CAD build for the part. Positions are in the model's coordinates, mm. Face numbers are marked on the shaded views. A direction names the side the tool comes from. Give positions to 0.01 mm unless a question says otherwise; leave off trailing zeros. Loops run counter-clockwise (first coordinate to the right, second up) from the corner with the lowest first, then second, coordinate; pieces in that order, holes last.
```python
from build123d import *

# Parameters (mm, degrees)
F1_DEPTH = 8


with BuildPart() as f1:
    # F0 (on Front) → F1 (new body)
    with BuildSketch(Plane.XZ):
        Polygon((-12, 6.928203), (-12, -6.928203), (0, -13.856406), (12, -6.928203), (12, 6.928203), (0, 13.856406), align=None)
    extrude(amount=F1_DEPTH)

    # F2 (on Right) → F3 (revolve)
    with BuildSketch(Plane.YZ):
        Polygon((1.602202, 3.686891), (0, 3.686891), (0, 0), (23.874549, 0), (23.874549, 3.686891), align=None)
    revolve(axis=Axis((0, 11.937275, 0), (0, 1, 0)))


solid = f1.part
```
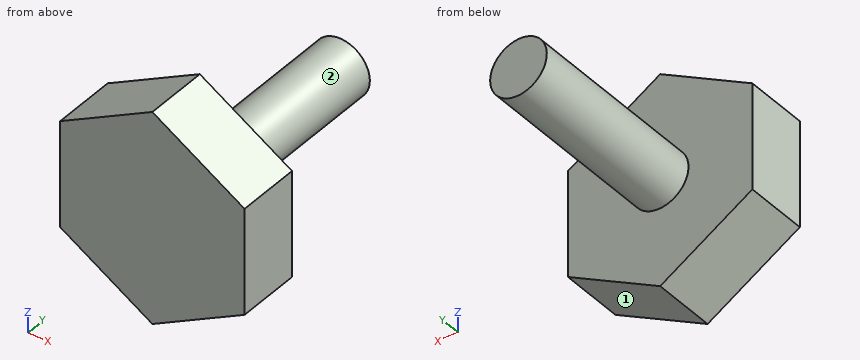
1. Saw through at A-A, the plane z = 0. List the corners of the cut face in (x, y), and give its area (3 significant figures).
Responses:
outline: (-12, -8) - (12, -8) - (12, 0) - (3.69, 0) - (3.69, 23.87) - (-3.69, 23.87) - (-3.69, 0) - (-12, 0) - close
area: 368 mm2
2. Drop flat-ended pins along their axis: pin 1 (12 mm diameter, centred on x = 2.5, z = 3, fed in from +Y); pin 2 (4 mm diameter, centred on x = 3.5, y = 2.5, fed in from +Z); pin 3 (5 mm diameter, centred on x = -2.5, y = 6, fed in from +Z). Give the stop position or say it passes through.
Responses:
pin 1: stops at y = 23.87
pin 2: stops at z = 3.37
pin 3: stops at z = 3.69
3. Saw through at C-C, the plane x = -5.25. List the corners of the cut face in (y, z), and give its area (3 significant figures).
Responses:
outline: (-8, -10.83) - (0, -10.83) - (0, 10.83) - (-8, 10.83) - close
area: 173 mm2
4. Probe line 1 along Y through (x, z) = (-8.75, 1.25); line 2 along Z through (x, y) = (-0.25, 8.5); line 3 along X through (y, z) = (6.5, -3). List the from-to ranges inside material, lowest first.
Responses:
line 1: y = -8 to 0
line 2: z = -3.68 to 3.68
line 3: x = -2.14 to 2.14
5. Saw through at D-D, the plane z = 11.75. List the corners of the cut face in (x, y).
Responses:
outline: (-3.65, -8) - (3.65, -8) - (3.65, 0) - (-3.65, 0) - close
6. Saw through at B-B, the plane x = -1.5. List the corners of the cut face in (y, z).
Responses:
outline: (-8, -12.99) - (0, -12.99) - (0, -3.37) - (23.87, -3.37) - (23.87, 3.37) - (0, 3.37) - (0, 12.99) - (-8, 12.99) - close
7. Tool access for the marked faces 1 and 2: list every direction of +Z, -Z, +X, -X, +Y, -Y with a clear straight run to the whole face (end or side of a thin tool).
Responses:
face 1: -Z, +X, +Y, -Y
face 2: +Y
